```python
from build123d import *

# Parameters (mm, degrees)
EXTRUDE1_DEPTH                                = 19.05
CSK_FOR_6_FLAT_HEAD_MACHINE_SCREW1_AT_2_COUNT = 2
CSK_FOR_6_FLAT_HEAD_MACHINE_SCREW1_AT_2_PITCH = 32.688625698
CSK_FOR_6_FLAT_HEAD_MACHINE_SCREW1_AT_3_COUNT = 2
CSK_FOR_6_FLAT_HEAD_MACHINE_SCREW1_AT_3_PITCH = 28.575
CSK_FOR_6_FLAT_HEAD_MACHINE_SCREW1_AT_4_COUNT = 2
CSK_FOR_6_FLAT_HEAD_MACHINE_SCREW1_AT_4_PITCH = 15.875
FILLET1_R                                     = 4.7752
SKETCH6_R                                     = 3.5433
SKETCH6_R_2                                   = 1.89865
BOSS_EXTRUDE1_DEPTH                           = 2.3876
CHAMFER1_SIZE                                 = 1.89865


with BuildPart() as part:
    # Sketch2 → Extrude1 (new, symmetric)
    with BuildSketch(Plane(origin=(0, 0, 0), x_dir=(0, 0, -1), z_dir=(1, 0, 0))):
        Polygon((-12.7, 2.3876), (-2.54, 2.3876), (-1.117284561, 1.1938), (1.117284561, 1.1938), (2.54, 2.3876), (12.7, 2.3876), (12.7, 0), (-12.7, 0), align=None)
    extrude(amount=EXTRUDE1_DEPTH, both=True)

    # Sketch5 → CSK for #6 Flat Head Machine Screw1 (revolve, cut)
    with BuildSketch(Plane(origin=(-14.2875, 2.3876, 7.9375), x_dir=(0, 0, 1), z_dir=(1, 0, 0))):
        Polygon((0, 0), (0, 2.3876), (1.89865, 2.3876), (1.89865, 1.891953401), (3.5433, 0), align=None)
    csk_for_6_flat_head_machine_screw1 = revolve(axis=Axis((-14.2875, 8.7376, 7.9375), (0, -1, 0)), mode=Mode.SUBTRACT)

    # CSK for #6 Flat Head Machine Screw1 at 2: CSK for #6 Flat Head Machine Screw1 ×2
    with Locations(*[Vector(0.8741572761215377, 0, -0.4856429311786321) * (i * CSK_FOR_6_FLAT_HEAD_MACHINE_SCREW1_AT_2_PITCH) for i in range(1, CSK_FOR_6_FLAT_HEAD_MACHINE_SCREW1_AT_2_COUNT)]):
        add(csk_for_6_flat_head_machine_screw1, mode=Mode.SUBTRACT)

    # CSK for #6 Flat Head Machine Screw1 at 3: CSK for #6 Flat Head Machine Screw1 ×2
    with Locations(*[(i * CSK_FOR_6_FLAT_HEAD_MACHINE_SCREW1_AT_3_PITCH, 0, 0) for i in range(1, CSK_FOR_6_FLAT_HEAD_MACHINE_SCREW1_AT_3_COUNT)]):
        add(csk_for_6_flat_head_machine_screw1, mode=Mode.SUBTRACT)

    # CSK for #6 Flat Head Machine Screw1 at 4: CSK for #6 Flat Head Machine Screw1 ×2
    with Locations(*[(0, 0, -i * CSK_FOR_6_FLAT_HEAD_MACHINE_SCREW1_AT_4_PITCH) for i in range(1, CSK_FOR_6_FLAT_HEAD_MACHINE_SCREW1_AT_4_COUNT)]):
        add(csk_for_6_flat_head_machine_screw1, mode=Mode.SUBTRACT)

    # Fillet1
    fillet1_edges = [part.edges().sort_by_distance(p)[0] for p in [
        (19.05, 1.1938, -12.7),
        (-19.05, 1.1938, 12.7),
        (19.05, 1.1938, 12.7),
        (-19.05, 1.1938, -12.7),
    ]]
    fillet(fillet1_edges, radius=FILLET1_R)

    # Sketch6 → Boss-Extrude1 (add)
    # profile 1 of 4: a face of its own
    with BuildSketch(Plane(origin=(0, 2.3876, 0), x_dir=(1, 0, 0), z_dir=(0, 1, 0))):
        with Locations((-14.2875, -7.9375)):
            Circle(SKETCH6_R)
        with Locations(Location((-14.2875, -7.9375, 0), (0, 0, 270))):
            Circle(SKETCH6_R_2, mode=Mode.SUBTRACT)
    # profile 2 of 4: a face of its own
    with BuildSketch(Plane(origin=(0, 2.3876, 0), x_dir=(1, 0, 0), z_dir=(0, 1, 0))):
        with Locations((-14.2875, 7.9375)):
            Circle(SKETCH6_R)
        with Locations(Location((-14.2875, 7.9375, 0), (0, 0, 270))):
            Circle(SKETCH6_R_2, mode=Mode.SUBTRACT)
    # profile 3 of 4: a face of its own
    with BuildSketch(Plane(origin=(0, 2.3876, 0), x_dir=(1, 0, 0), z_dir=(0, 1, 0))):
        with Locations((14.2875, -7.9375)):
            Circle(SKETCH6_R)
        with Locations(Location((14.2875, -7.9375, 0), (0, 0, 270))):
            Circle(SKETCH6_R_2, mode=Mode.SUBTRACT)
    # profile 4 of 4: a face of its own
    with BuildSketch(Plane(origin=(0, 2.3876, 0), x_dir=(1, 0, 0), z_dir=(0, 1, 0))):
        with Locations((14.2875, 7.9375)):
            Circle(SKETCH6_R)
        with Locations(Location((14.2875, 7.9375, 0), (0, 0, 270))):
            Circle(SKETCH6_R_2, mode=Mode.SUBTRACT)
    extrude(amount=-BOSS_EXTRUDE1_DEPTH)

    # Chamfer1
    chamfer1_edges = [part.edges().sort_by_distance(p)[0] for p in [
        (-14.2875, 0, -9.83615),
        (14.2875, 0, 6.03885),
        (14.2875, 0, -9.83615),
        (-14.2875, 0, 6.03885),
    ]]
    chamfer(chamfer1_edges, length=CHAMFER1_SIZE)


solid = part.part
```
Design review of the part built by this model. Coordinates are the model's own, in mm. A direction names the side the tool comes from. Coordinates: 2 decimals unless noted, no trailing zeros. Order: outer loops, then holes, each group sorted by start corner. A loop starts at its lowest first (then second) coordinate and runs counter-clockwise, first axis right, second up. Notation, with made-up numbers: M 82.25,77.5 L 95.25,77.5 A27 cw 95.25,108.5 Z; hole C 72.5,-3.5 d1. An arc over 180 degrees is marked long. Answer as a JSON object with one key per item and string values. Group by question number.
1) Tool access review of faces 1 (the cylindrical face through (17.61, 1.21, 11.34)), 2 (the flat face through (0.27, 1.8, 1.84)): name each direction out of +Z, -Z, +X, -X, +Y, -Y from which nothing blocks a thin tool from reaching the whole face with its end or side.
2) Add section C-C, the plane x = 13.5. Count the separate pieces of the cut face and the enclosed holes in it, then the cut area to 3 significant figures.
3) Add section A-A, the plane x = 0. Write out the cut boundary in (y, z), then the cut area to 3 significant figures.
4) Add section B-B, the plane y = 0.7. Write out the cut boundary in (x, z), then the cut area to 3 significant figures.
5) Wall thickness on L1, parallel to X at y = 1, z = -10.25; L2, parallel to X at y = 1.05, z = -7; L3, parallel to Y at x = 7.5, z = 1: over which ranges is each line inside the solid? List them lowest first.
6) Mouldability with a two-part tool opening along X and no side actions: class faces 3 (the conical face through (-14.89, 1.78, 9.86)), 4 (the flat face through (0.267, 1.782, -1.819)), 5 (the cylindrical face through (-17.61, 1.21, 11.34)) as pulls with the +X half, pulls with the -X half, needs draft (parallel to the pull), parting line crosses it, or undercut.
7) For pin 1 (6 mm diameter, centred on x = 14.29, z = -7.94, fed in from -Y); pin 2 (3 mm diameter, centred on x = -14.29, z = 7.94, fed in from +Y); pin 3 (2.5 mm diameter, centred on x = -3, z = 0, fed in from +Y); pin 4 (4.5 mm diameter, centred on x = 14.29, z = 7.94, fed in from -Y), all flat-tipped, find the tip position at first contact; note any pin that passes through.
Computed values:
{
 "1": {"face 1": "+Z, +X, +Y, -Y", "face 2": "+X, -X, +Y"},
 "2": {"separate pieces": "3", "enclosed holes": "0", "area": "32.2 mm^2"},
 "3": {"outline": "M 0,-12.7 L 2.39,-12.7 L 2.39,-2.54 L 1.19,-1.12 L 1.19,1.12 L 2.39,2.54 L 2.39,12.7 L 0,12.7 Z", "area": "56.3 mm^2"},
 "4": {"outline": "M -19.05,-7.92 A4.78 ccw -14.27,-12.7 L 14.27,-12.7 A4.78 ccw 19.05,-7.92 L 19.05,7.92 A4.78 ccw 14.27,12.7 L -14.27,12.7 A4.78 ccw -19.05,7.92 Z; hole C -14.29,-7.94 d6.19; hole C -14.29,7.94 d6.19; hole C 14.29,-7.94 d6.19; hole C 14.29,7.94 d6.19", "area": "828 mm^2"},
 "5": {"L1": "x = -18.45 to -15.86, -12.71 to 12.71, 15.86 to 18.45", "L2": "x = -19.05 to -16.87, -11.71 to 11.71, 16.87 to 19.05", "L3": "y = 0 to 1.19"},
 "6": {"face 3": "undercut", "face 4": "needs draft", "face 5": "pulls with the -X half"},
 "7": {"pin 1": "stops at y = 0.79", "pin 2": "passes through", "pin 3": "stops at y = 1.31", "pin 4": "stops at y = 1.54"}
}
